Input: part model. Units: mm. Frame: model coordinates. A direction names the side the tool comes from. Give positions to 0.01 mm unless a question says otherwise; leave off trailing zeros. Loops run counter-clockwise (first coordinate to the right, second up) from the corner with the lowest first, then second, coordinate; pieces in that order, holes last. Notation, with made-up numbers: (75.5, 31) -> (112.5, 31) arc R25 ccw to (112.5, 54) -> close; hole circle Ø7 at (35.25, 4.25). An arc over 180 degrees is marked (long way). Use CSV: the item, a comma, the result in double quotes.
```python
from build123d import *

# Parameters (mm, degrees)
SKETCH1_R           = 56
SKETCH1_R_2         = 4.05
BOSS_EXTRUDE1_DEPTH = 3


with BuildPart() as part:
    # Sketch1 → Boss-Extrude1 (new body)
    with BuildSketch(Plane.XY):
        Circle(SKETCH1_R)
        with Locations((-23.5, 40.703193978)):
            Circle(SKETCH1_R_2, mode=Mode.SUBTRACT)
        with Locations((-23.5, -40.703193978)):
            Circle(SKETCH1_R_2, mode=Mode.SUBTRACT)
        with Locations((47, 0)):
            Circle(SKETCH1_R_2, mode=Mode.SUBTRACT)
        with BuildLine():
            Line((-20.603621104, 31.05), (-35.603621104, 31.05))
            ThreePointArc((-35.603621104, 31.05), (-37.724941448, 30.171320344), (-38.603621104, 28.05))
            Line((-38.603621104, 28.05), (-38.603621104, 2.45))
            Line((-38.603621104, 2.45), (-38.603621104, -28.05))
            ThreePointArc((-38.603621104, -28.05), (-37.724941448, -30.171320344), (-35.603621104, -31.05))
            Line((-35.603621104, -31.05), (-20.603621104, -31.05))
            ThreePointArc((-20.603621104, -31.05), (-17.018844263, -30.657863153), (-13.603621104, -29.5))
            Line((-13.603621104, -29.5), (-13.603621104, 29.5))
            ThreePointArc((-13.603621104, 29.5), (-17.018844263, 30.657863153), (-20.603621104, 31.05))
        make_face(mode=Mode.SUBTRACT)
    extrude(amount=BOSS_EXTRUDE1_DEPTH)


solid = part.part
```
1) Section query D-D (z = 0.75). Return loops of the section in (x, y), then the cut area to 3 significant figures.
From the geometry:
outline,"circle Ø112 at (0, 0); hole (-38.6, -28.05) arc R3 ccw to (-35.6, -31.05) -> (-20.6, -31.05) arc R16.58 ccw to (-13.6, -29.5) -> (-13.6, 29.5) arc R16.58 ccw to (-20.6, 31.05) -> (-35.6, 31.05) arc R3 ccw to (-38.6, 28.05) -> close; hole circle Ø8.1 at (-23.5, -40.7); hole circle Ø8.1 at (-23.5, 40.7); hole circle Ø8.1 at (47, 0)"
area,"8,160 mm^2"
2) Section query B-B (y = -38). Return loops of the section in (x, z).
From the geometry:
outline,"(-41.13, 0) -> (-26.52, 0) -> (-26.52, 3) -> (-41.13, 3) -> close; (-20.48, 0) -> (41.13, 0) -> (41.13, 3) -> (-20.48, 3) -> close"
3) Contact query for flat-ended pins moving along their axis: pin 1 (0.9 mm diameter, centred on x = -30, z = 2, fed in from +Y); pin 2 (1.5 mm diameter, centred on x = 8.5, z = 1.5, fed in from -Y). Output: stop coordinate, or through.
From the geometry:
pin 1,"stops at y = 47.57"
pin 2,"stops at y = -55.46"
4) Reachability of faces 5 (the cylindrical face through (-16.969, 30.647, 1.479)), 6 (the flat face through (12, 1, 0)) from +Z, -Z, +X, -X, +Y, -Y: full face, straight path, thin tool, end or side. Return the list, or none.
From the geometry:
face 5,"+Z, -Z"
face 6,"-Z, +X, -X, +Y, -Y"
5) Mould query, pull axis Y, two halves, no side actions, for faces 1 (the cylindrical face through (43.786, -2.464, 1.479)), 2 (the flat face through (-28, 31.05, 1)), 3 (the flat face through (12, 1, 3)), 4 (the cylindrical face through (51.73, -21.45, 1.48)). Classes: pulls with the +Y half, pulls with the -Y half, needs draft (parallel to the pull), parting line crosses it, or undercut.
From the geometry:
face 1,"undercut"
face 2,"undercut"
face 3,"needs draft"
face 4,"parting line crosses it"
6) Ray query, line 1 (Y direction, x = -23.5, z = 0.75); line 2 (X direction, y = -1.5, z = 0.4). Return the intervals inside material, ascending.
From the geometry:
line 1,"y = -50.83 to -44.75, -36.65 to -31.05, 31.05 to 36.65, 44.75 to 50.83"
line 2,"x = -55.98 to -38.6, -13.6 to 43.24, 50.76 to 55.98"
7) Section query A-A (y = 0). Return loops of the section in (x, z).
From the geometry:
outline,"(-56, 0) -> (-38.6, 0) -> (-38.6, 3) -> (-56, 3) -> close; (-13.6, 0) -> (42.95, 0) -> (42.95, 3) -> (-13.6, 3) -> close; (51.05, 0) -> (56, 0) -> (56, 3) -> (51.05, 3) -> close"
8) Section query C-C (x = 47). Return loops of the section in (y, z), then the cut area to 3 significant figures.
From the geometry:
outline,"(-30.45, 0) -> (-4.05, 0) -> (-4.05, 3) -> (-30.45, 3) -> close; (4.05, 0) -> (30.45, 0) -> (30.45, 3) -> (4.05, 3) -> close"
area,"158 mm^2"
